```python
from build123d import *

# Parameters (mm, degrees)
SKETCH1_W           = 50
SKETCH1_H           = 50
BOSS_EXTRUDE1_DEPTH = 3.5
SKETCH2_R           = 3.75
BOSS_EXTRUDE2_DEPTH = 16
SKETCH3_R           = 3.5
CUT_EXTRUDE2_DEPTH  = 19.5
SKETCH4_W           = 40
SKETCH4_H           = 9.367616821
CUT_EXTRUDE3_DEPTH  = 19.5


with BuildPart() as part:
    # Sketch1 → Boss-Extrude1 (new body)
    with BuildSketch(Plane.XY):
        with Locations((25, 25)):
            Rectangle(SKETCH1_W, SKETCH1_H)
    extrude(amount=BOSS_EXTRUDE1_DEPTH)

    # Sketch2 → Boss-Extrude2 (add)
    with BuildSketch(Plane.XY.offset(3.5)):
        Circle(SKETCH2_R)
        with Locations(Location((50, 0, 0), (0, 0, 180))):
            Circle(SKETCH2_R)
    extrude(amount=BOSS_EXTRUDE2_DEPTH)

    # Sketch3 → Cut-Extrude2 (cut)
    with BuildSketch(Plane.XY.offset(19.5)):
        Circle(SKETCH3_R)
        with Locations((50, 0)):
            Circle(SKETCH3_R)
    extrude(amount=-CUT_EXTRUDE2_DEPTH, mode=Mode.SUBTRACT)

    # Sketch4 → Cut-Extrude3 (cut)
    with BuildSketch(Plane.XY.offset(3.5)):
        with Locations((25, 40.31619159)):
            Rectangle(SKETCH4_W, SKETCH4_H)
    extrude(amount=-CUT_EXTRUDE3_DEPTH, mode=Mode.SUBTRACT)


solid = part.part
```
Source: CAD feature listing. Evaluate the final solid. Frame: model axes, mm. A direction names the side the tool comes from. Give positions to 0.01 mm unless a question says otherwise; leave off trailing zeros. Loops run counter-clockwise (first coordinate to the right, second up) from the corner with the lowest first, then second, coordinate; pieces in that order, holes last. Notation, with made-up numbers: (68, 55.5) - (72, 55.5) arc R30 ccw to (72, 90.5) - close; hole circle Ø2 at (-37.5, 80.25). An arc over 180 degrees is marked (long way). Use CSV: the item, a comma, the result in double quotes. Start each with the question number.
1. Section A-A (y = 41.5). Output: boundary loops of the cut face in (x, z), then the cut area to 3 significant figures.
2. Pin query (flat end, axial travel): pin 1 (10 mm diameter, centred on x = 13.5, z = 11.5, fed in from +Y); pin 2 (1 mm diameter, centred on y = 38.5, z = 1, fed in from +X); pin 3 (8 mm diameter, centred on x = 9, y = 18.5, fed in from +Z); pin 4 (4 mm diameter, centred on x = -1.5, y = 0.5, fed in from -Z). Return the tip coordinate at first contact, or that it passes through.
3. Section C-C (x = 33.5). Output: boundary loops of the cut face in (y, z), then the cut area to 3 significant figures.
4. Section B-B (z = 5). Output: boundary loops of the cut face in (x, y), then the cut area to 3 significant figures.
5. Section D-D (y = 34.5). Output: boundary loops of the cut face in (x, z), then the cut area to 3 significant figures.
6. Reachability of faces 4 (the flat face through (25, 20, 3.5)), 5 (the cylindrical face through (46.423, -1.126, 11.388)), 6 (the flat face through (25, 45, 2)) from +Z, -Z, +X, -X, +Y, -Y: full face, straight path, thin tool, end or side. Return the list, or none.
7. Draft query along X for faces 1 (the flat face through (25, 0, 2)), 2 (the cylindrical face through (-3.746, 0.165, 11.388)), 3 (the flat face through (50, 26, 2)). Return one class per face: +X half, -X half, draft (parallel to the pull), parting line (faces both ways), or undercut.
8. Ray query, L1, parallel to Y at x = 0, z = 6.75; L2, parallel to Y at x = 20, z = 3.25; L3, parallel to X at y = 34, z = 2.5. Return the intervals inside material, ascending.
Response:
1,outline,"(0, 0) - (5, 0) - (5, 3.5) - (0, 3.5) - close; (45, 0) - (50, 0) - (50, 3.5) - (45, 3.5) - close"
1,area,"35.0 mm²"
2,pin 1,"through"
2,pin 2,"x = 50"
2,pin 3,"z = 3.5"
2,pin 4,"z = 3.5"
3,outline,"(0, 0) - (35.63, 0) - (35.63, 3.5) - (0, 3.5) - close; (45, 0) - (50, 0) - (50, 3.5) - (45, 3.5) - close"
3,area,"142 mm²"
4,outline,"circle Ø7.5 at (0, 0); circle Ø7.5 at (50, 0); hole circle Ø7 at (0, 0); hole circle Ø7 at (50, 0)"
4,area,"11.4 mm²"
5,outline,"(0, 0) - (50, 0) - (50, 3.5) - (0, 3.5) - close"
5,area,"175 mm²"
6,face 4,"+Z, +Y"
6,face 5,"+Z"
6,face 6,"+Z, -Z"
7,face 1,"draft"
7,face 2,"undercut"
7,face 3,"+X half"
8,L1,"-3.75 to -3.5, 3.5 to 3.75"
8,L2,"0 to 35.63, 45 to 50"
8,L3,"0 to 50"
